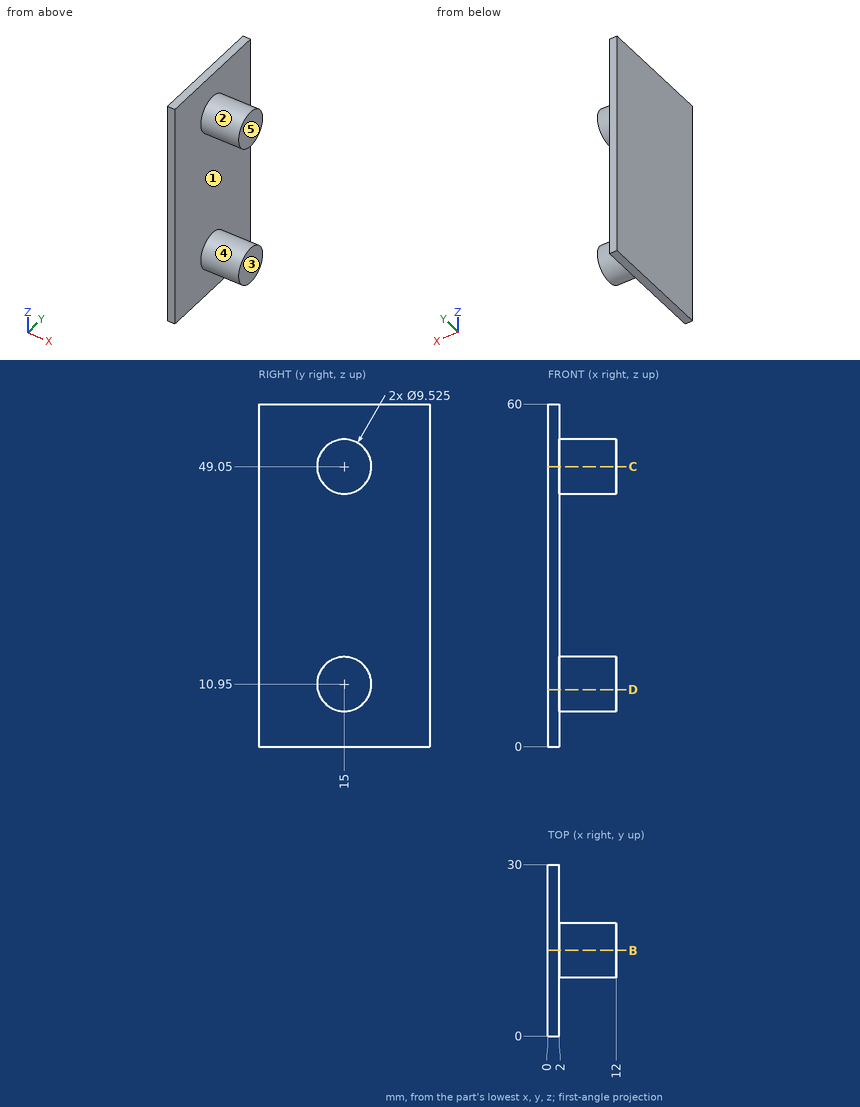
Geometry: see drawing. Coordinates: mm, zero at the bounding-box minimum. A direction names the side the tool comes from. Give positions to 0.01 mm unless a question says otherwise; leave off trailing zeros. Loops run counter-clockwise (first coordinate to the right, second up) from the corner with the lowest first, then second, coordinate; pieces in that order, holes last. Notation, with made-up numbers: (39.25, 66.5) - (47.25, 66.5) arc R31 ccw to (47.25, 101.5) - close; hole circle Ø9 at (45, 63). An arc over 180 degrees is marked (long way). Use CSV: the item, a comma, the result in double quotes. Start each with the question number.
1. Section C-C (z = 49.05). Output: boundary loops of the cut face in (x, y).
2. Draft query along Z for the marked faces 1, 2 and 3. Return one class per face: +Z half, -Z half, draft (parallel to the pull), parting line (faces both ways), or undercut.
3. Reachability of the marked faces 4 and 5 from +Z, -Z, +X, -X, +Y, -Y: full face, straight path, thin tool, end or side. Return the list, or none.
4. Section B-B (y = 15). Output: boundary loops of the cut face in (x, z), then the cut area to 4 significant figures.
5. Ray query, L1, parallel to X at y = 22.75, z = 56; L2, parallel to Y at x = 4.25, z = 11; L3, parallel to Z at x = 4.5, y = 17.75. Return the intervals inside material, ascending.
6. Pin query (flat end, axial travel): pin 1 (1.5 mm diameter, centred on y = 12.5, z = 39, fed in from -X); pin 2 (1.5 mm diameter, centred on x = 4, y = 17, fed in from +Z). Return the tip coordinate at first contact, or that it passes through.
7. Section D-D (z = 10). Output: boundary loops of the cut face in (x, y), then the cut area to 3 significant figures.
Response:
1,outline,"(0, 0) - (2, 0) - (2, 10.24) - (12, 10.24) - (12, 19.76) - (2, 19.76) - (2, 30) - (0, 30) - close"
2,face 1,"undercut"
2,face 2,"undercut"
2,face 3,"draft"
3,face 4,"+X"
3,face 5,"+Z, -Z, +X, +Y, -Y"
4,outline,"(0, 0) - (2, 0) - (2, 6.19) - (12, 6.19) - (12, 15.71) - (2, 15.71) - (2, 44.29) - (12, 44.29) - (12, 53.81) - (2, 53.81) - (2, 60) - (0, 60) - close"
4,area,"310.5 mm²"
5,L1,"0 to 2"
5,L2,"10.24 to 19.76"
5,L3,"7.06 to 14.84, 45.16 to 52.94"
6,pin 1,"x = 0"
6,pin 2,"z = 53.65"
7,outline,"(0, 0) - (2, 0) - (2, 10.33) - (12, 10.33) - (12, 19.67) - (2, 19.67) - (2, 30) - (0, 30) - close"
7,area,"153 mm²"
